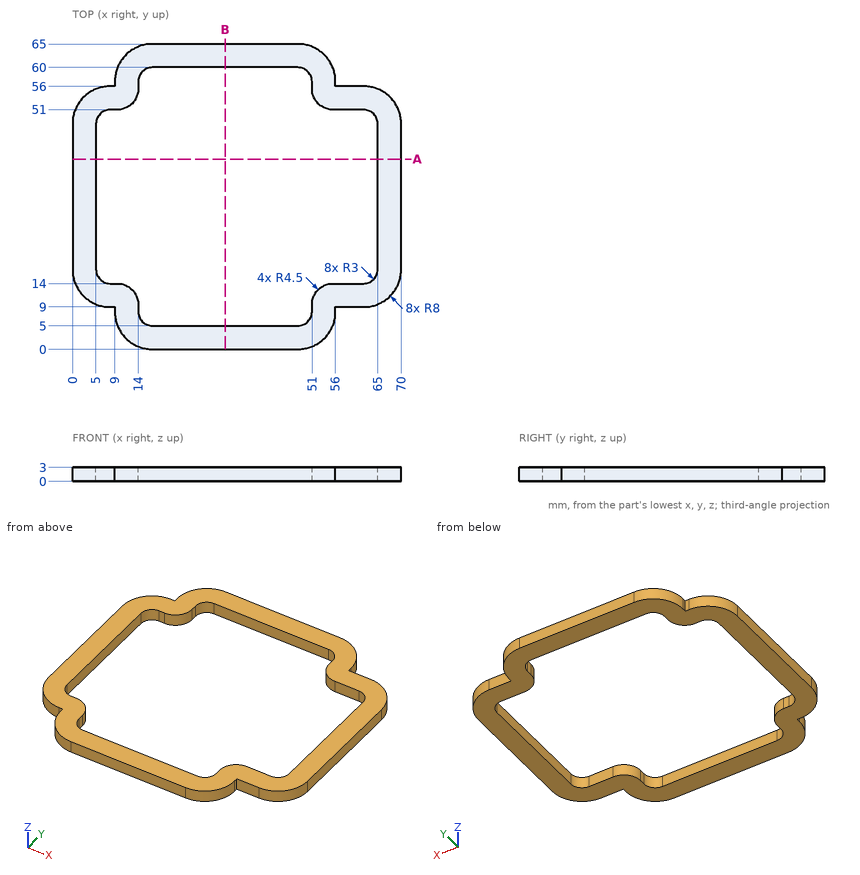
Design review of the part shown in the three views and the two pictorial views. Dimensions are in mm from the part's minimum x, y and z. Give positions to 0.01 mm unless a question says otherwise; leave off trailing zeros. Loops run counter-clockwise (first coordinate to the right, second up) from the corner with the lowest first, then second, coordinate; pieces in that order, holes last. Notation, with made-up numbers: M 0,37.25 L 21,37.25 A24 ccw 21,60.25 Z; hole C 80,-26.75 d7. An arc over 180 degrees is marked long. Answer as a JSON object with one key per item and string values. Group by question number.
Q1. Add section A-A on y = 40.5. Give the boundary of the cut face in (x, z), and give its area (3 significant figures).
Q2. Insertion check: P1, Ø0.8, axis at y = 8.5, z = 2, coming from the +X side; P2, Ø1.2, axis at y = 9, z = 2, coming from the -X side; P3, Ø0.9, axis at x = 60.5, z = 1, coming from the +Y side. Each pin has a flat end and moves straight along its axis. Give the tip position at first contact, or say it passes through.
Q3. For probe 1 along Y at (x, z) = (59, 2); probe 2 along X at (y, z) = (40, 0.75); probe 3 along Y at (x, z) = (26.5, 1.75), list the stretches that pass through material, from the lowest coordinate up. Write a range as [from, to].
Q4. Add section B-B on x = 32.5. Give the boundary of the cut face in (y, z), and give its area (3 significant figures).
Checked values:
{
 "1": {"outline": "M 0,0 L 5,0 L 5,3 L 0,3 Z; M 65,0 L 70,0 L 70,3 L 65,3 Z", "area": "30.0 mm²"},
 "2": {"P1": "x = 56", "P2": "x = 4.96", "P3": "y = 56"},
 "3": {"probe 1": "[9, 14], [51, 56]", "probe 2": "[0, 5], [65, 70]", "probe 3": "[0, 5], [60, 65]"},
 "4": {"outline": "M 0,0 L 5,0 L 5,3 L 0,3 Z; M 60,0 L 65,0 L 65,3 L 60,3 Z", "area": "30.0 mm²"}
}
